from build123d import *

# Parameters (mm, degrees)
SKETCH1_R           = 0.75
BOSS_EXTRUDE1_DEPTH = 1
SKETCH2_R           = 3.67931812
BOSS_EXTRUDE2_DEPTH = 5
SKETCH2_3_R         = 1.5
CUT_EXTRUDE1_DEPTH  = 0.5
SKETCH1_2_R         = 0.75
CUT_EXTRUDE2_DEPTH  = 19.333027078
SKETCH3_R           = 2.355
CUT_EXTRUDE3_DEPTH  = 2


with BuildPart() as part:
    # Sketch1 → Boss-Extrude1 (new body)
    with BuildSketch(Plane(origin=(0, 0, 0), x_dir=(1, 0, 0), z_dir=(0, 1, 0))):
        with BuildLine():
            Line((-2.49119588, 14.959626071), (-3.608885156, 1.677008569))
            ThreePointArc((-3.608885156, 1.677008569), (-3.67931812, 0), (-3.608885156, -1.677008569))
            Line((-3.608885156, -1.677008569), (-2.49119588, -14.959626071))
            ThreePointArc((-2.49119588, -14.959626071), (0, -17.25), (2.49119588, -14.959626071))
            Line((2.49119588, -14.959626071), (3.608885156, -1.677008569))
            ThreePointArc((3.608885156, -1.677008569), (3.67931812, 0), (3.608885156, 1.677008569))
            Line((3.608885156, 1.677008569), (2.49119588, 14.959626071))
            ThreePointArc((2.49119588, 14.959626071), (0, 17.25), (-2.49119588, 14.959626071))
        make_face()
        with Locations(Location((0, 14.75, 0), (0, 0, 270))):
            Circle(SKETCH1_R, mode=Mode.SUBTRACT)
        with Locations(Location((0, 12.75, 0), (0, 0, 270))):
            Circle(SKETCH1_R, mode=Mode.SUBTRACT)
        with Locations(Location((0, 10.75, 0), (0, 0, 270))):
            Circle(SKETCH1_R, mode=Mode.SUBTRACT)
        with Locations(Location((0, 8.75, 0), (0, 0, 270))):
            Circle(SKETCH1_R, mode=Mode.SUBTRACT)
        with Locations(Location((0, 6.75, 0), (0, 0, 270))):
            Circle(SKETCH1_R, mode=Mode.SUBTRACT)
        with Locations(Location((0, 4.75, 0), (0, 0, 270))):
            Circle(SKETCH1_R, mode=Mode.SUBTRACT)
        with Locations(Location((0, 0, 0), (0, 0, 270))):
            Circle(SKETCH1_R, mode=Mode.SUBTRACT)
        with Locations(Location((0, -4.75, 0), (0, 0, 90))):
            Circle(SKETCH1_R, mode=Mode.SUBTRACT)
        with Locations(Location((0, -6.75, 0), (0, 0, 90))):
            Circle(SKETCH1_R, mode=Mode.SUBTRACT)
        with Locations(Location((0, -8.75, 0), (0, 0, 90))):
            Circle(SKETCH1_R, mode=Mode.SUBTRACT)
        with Locations(Location((0, -10.75, 0), (0, 0, 90))):
            Circle(SKETCH1_R, mode=Mode.SUBTRACT)
        with Locations(Location((0, -12.75, 0), (0, 0, 90))):
            Circle(SKETCH1_R, mode=Mode.SUBTRACT)
        with Locations(Location((0, -14.75, 0), (0, 0, 90))):
            Circle(SKETCH1_R, mode=Mode.SUBTRACT)
    extrude(amount=BOSS_EXTRUDE1_DEPTH)

    # Sketch2 → Boss-Extrude2 (add)
    with BuildSketch(Plane.XZ):
        with Locations(Location((0, 0, 0), (0, 0, 270))):
            Circle(SKETCH2_R)
    extrude(amount=-BOSS_EXTRUDE2_DEPTH)

    # Sketch2_3 → Cut-Extrude1 (cut)
    with BuildSketch(Plane.XZ):
        with Locations(Location((0, 0, 0), (0, 0, 270))):
            Circle(SKETCH2_3_R)
    extrude(amount=-CUT_EXTRUDE1_DEPTH, mode=Mode.SUBTRACT)

    # Sketch1_2 → Cut-Extrude2 (cut, through all)
    with BuildSketch(Plane(origin=(0, 0, 0), x_dir=(1, 0, 0), z_dir=(0, 1, 0))):
        with Locations(Location((0, 0, 0), (0, 0, 90))):
            Circle(SKETCH1_2_R)
    extrude(amount=CUT_EXTRUDE2_DEPTH, mode=Mode.SUBTRACT)

    # Sketch3 → Cut-Extrude3 (cut)
    with BuildSketch(Plane(origin=(0, 5, 0), x_dir=(1, 0, 0), z_dir=(0, 1, 0))):
        with Locations(Location((0, 0, 0), (0, 0, 270))):
            Circle(SKETCH3_R)
    extrude(amount=-CUT_EXTRUDE3_DEPTH, mode=Mode.SUBTRACT)


solid = part.part
The listing builds one solid part. Answer for the finished solid, in the listing's coordinates (mm). A direction names the side the tool comes from. Coordinates: 2 decimals unless noted, no trailing zeros. Loops run counter-clockwise (first coordinate to the right, second up) from the corner with the lowest first, then second, coordinate; pieces in that order, holes last. Notation, with made-up numbers: (47.25, 34) -> (91.25, 34) arc R29 ccw to (91.25, 62) -> close; hole circle Ø9 at (30.5, 82.25). An arc over 180 degrees is marked (long way). Write item = value, one per line. Start each with the question number.
1) A cutting plane is placed at C-C (y = 2.4). Give the vertices of the cut face in (x, z).
2) Straight lines are drawn through the part: line 1 (Y direction, x = 2.5, z = 14); line 2 (X direction, y = 3.85, z = 0) (3 decimals); line 3 (X direction, y = 0.6, z = 4.75). For each, find the intervals that lie inside material, in ascending order. Write a range as from..to.
3) The mould has two halves that part along Z. Classify faces 1 (the face through (-3.59, 2.97, 0.8)), 2 (the face through (1, 0.5, 0)), 3 (the face through (-0.05, 0.49, 17.25)), 4 (the face through (-2.4, 5, -0.8)): released by +Z, released by -Z, zero draft, split by the parting line, or undercut.
4) A cutting plane is placed at D-D (z = -4.75). Give the vertices of the cut face in (x, y).
5) A cutting plane is placed at B-B (x = 0). Count the separate pieces of the cut face and the enclosed holes in it, then the cut area to 3 significant figures.
6) A tool of negligible diameter and unlimited length cuts with its end or side. For faces 5 (the face through (-2.3, 4, -0.5)), 6 (the face through (-3.058, 0.493, 8.225)), from which of +Z, -Z, +X, -X, +Y, -Y can it reach the whole face along a straight path? Write none if from no direction.
7) A cutting plane is placed at A-A (z = -8.75). Give the vertices of the cut face in (x, y), then the cut area to 3 significant figures.
8) Given pin 1 Ø0.9 at (x, z) = (0, -12.75) entering from -Y; pin 2 Ø3 at (x, y) = (2.5, 1.5) entering from -Z; pin 3 Ø1.7 at (x, z) = (0, -10.75) entering from +Y; pin 4 Ø1.4 at (x, z) = (0.5, 0) entering from +Y, each flat-ended and moving along its own axis, determine where each tip first touches the part or whether it passes through.
Responses:
q1.outline = circle Ø7.36 at (0, 0); hole circle Ø1.5 at (0, 0)
q2.line_1 = 0..1
q2.line_2 = -3.679..-2.355, 2.355..3.679
q2.line_3 = -3.35..-0.75, 0.75..3.35
q3.face_1 = split by the parting line
q3.face_2 = undercut
q3.face_3 = released by +Z
q3.face_4 = zero draft
q4.outline = (-3.35, 0) -> (-0.75, 0) -> (-0.75, 1) -> (-3.35, 1) -> close; (0.75, 0) -> (3.35, 0) -> (3.35, 1) -> (0.75, 1) -> close
q5.separate_pieces = 14
q5.enclosed_holes = 0
q5.area = 31.3 mm²
q6.face_5 = +Y
q6.face_6 = +Z, -X, +Y, -Y
q7.outline = (-3.01, 0) -> (-0.75, 0) -> (-0.75, 1) -> (-3.01, 1) -> close; (0.75, 0) -> (3.01, 0) -> (3.01, 1) -> (0.75, 1) -> close
q7.area = 4.53 mm²
q8.pin_1 = through
q8.pin_2 = -17
q8.pin_3 = 1
q8.pin_4 = 3
